Design review of the part built by this model. Coordinates are the model's own, in mm. Face numbers are marked on the shaded views. Coordinates: 2 decimals unless noted, no trailing zeros. Answer in a Markdown table with one row per item.
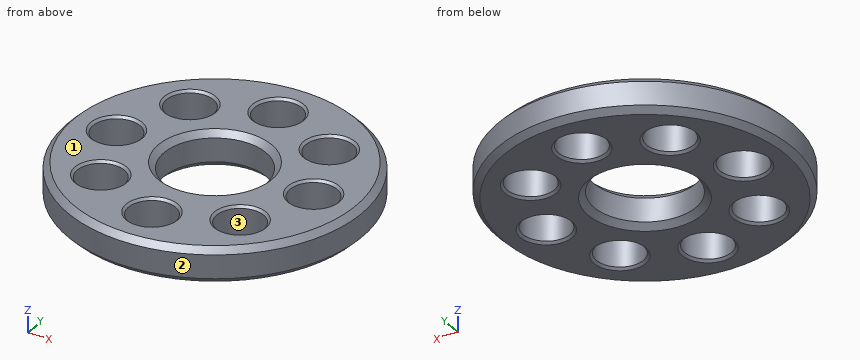
```python
from build123d import *

# Parameters (mm, degrees)
F0_R     = 31.75
F0_R_2   = 5.08
F0_R_3   = 11.000003
F1_DEPTH = 7.62
F2_SIZE  = 1.27
F3_SIZE  = 1.27
F4_SIZE  = 0.508


with BuildPart() as f1:
    # F0 (on Top) → F1 (new body)
    with BuildSketch(Plane.XY):
        Circle(F0_R)
        with Locations((-15.266435, -15.266435)):
            Circle(F0_R_2, mode=Mode.SUBTRACT)
        with Locations((0, -21.59)):
            Circle(F0_R_2, mode=Mode.SUBTRACT)
        with Locations((15.266435, -15.266435)):
            Circle(F0_R_2, mode=Mode.SUBTRACT)
        with Locations((-21.59, 0)):
            Circle(F0_R_2, mode=Mode.SUBTRACT)
        with Locations((-15.266435, 15.266435)):
            Circle(F0_R_2, mode=Mode.SUBTRACT)
        Circle(F0_R_3, mode=Mode.SUBTRACT)
        with Locations((15.266435, 15.266435)):
            Circle(F0_R_2, mode=Mode.SUBTRACT)
        with Locations((21.59, 0)):
            Circle(F0_R_2, mode=Mode.SUBTRACT)
        with Locations((0, 21.59)):
            Circle(F0_R_2, mode=Mode.SUBTRACT)
    extrude(amount=F1_DEPTH)

    # F2
    f2_edges = [f1.edges().sort_by_distance(p)[0] for p in [
        (-31.75, 0, 7.62),
        (-11.000003, 0, 7.62),
    ]]
    chamfer(f2_edges, length=F2_SIZE)

    # F3
    f3_edges = [f1.edges().sort_by_distance(p)[0] for p in [
        (-31.75, 0, 0),
        (-11.000003, 0, 0),
    ]]
    chamfer(f3_edges, length=F3_SIZE)

    # F4
    f4_edges = [f1.edges().sort_by_distance(p)[0] for p in [
        (-5.08, -21.59, 0),
        (20.346435, -15.266435, 3.81),
        (10.186435, -15.266435, 0),
        (10.186435, -15.266435, 7.62),
        (5.08, -21.59, 3.81),
        (-5.08, -21.59, 7.62),
        (-10.186435, -15.266435, 3.81),
        (-20.346435, -15.266435, 0),
        (-20.346435, -15.266435, 7.62),
        (-16.51, 0, 3.81),
        (-26.67, 0, 0),
        (-26.67, 0, 7.62),
        (-10.186435, 15.266435, 3.81),
        (-20.346435, 15.266435, 0),
        (-20.346435, 15.266435, 7.62),
        (5.08, 21.59, 3.81),
        (-5.08, 21.59, 0),
        (-5.08, 21.59, 7.62),
        (20.346435, 15.266435, 3.81),
        (10.186435, 15.266435, 0),
        (10.186435, 15.266435, 7.62),
        (16.51, 0, 0),
        (26.67, 0, 3.81),
        (16.51, 0, 7.62),
    ]]
    chamfer(f4_edges, length=F4_SIZE)


solid = f1.part
```
(1) For pin 1 (2 mm diameter, centred on y = -23, z = 6, fed in from +X), flat-tipped, find the tip position at first contact; note if it passes through.
Evaluation:
| item | result |
|---|---|
| pin 1 | stops at x = 22.89 |
(2) Draft analysis for pull direction Y (two halves, no side actions). For the marked faces 1, 2 and 3, state which applies: pulls with the +Y half, pulls with the -Y half, needs draft (parallel to the pull), parting line crosses it, or undercut.
Evaluation:
| item | result |
|---|---|
| face 1 | needs draft |
| face 2 | parting line crosses it |
| face 3 | undercut |
(3) To check wall thickness, follow probe 1 along Y at (x, z) = (0, 4); probe 2 along Y at (x, z) = (3.5, 0.75); probe 3 along X at (y, z) = (-13, 7.25). State the ranges of each line that lie inside material, in increasing order.
Evaluation:
| item | result |
|---|---|
| probe 1 | y = -31.75 to -26.67, -16.51 to -11, 11 to 16.51, 26.67 to 31.75 |
| probe 2 | y = -31.03 to -25.27, -17.91 to -10.98, 10.98 to 17.91, 25.27 to 31.03 |
| probe 3 | x = -27.98 to -19.97, -10.57 to 10.57, 19.97 to 27.98 |
(4) Take a section at A-A on y = 0. Count the separate pieces of the cut face and the enclosed holes in it, and give its area (3 significant figures).
Evaluation:
| item | result |
|---|---|
| separate pieces | 4 |
| enclosed holes | 0 |
| area | 154 mm² |
